The figure shows three views and two pictorial views of one solid part (mm, origin at its lowest corner). Answer the questions. Round coordinates to 2 decimals unless told otherwise and drop trailing zeros. Order: outer loops, then holes, each group sorted by start corner. A loop starts at its lowest first (then second) coordinate and runs counter-clockwise, first axis right, second up. Notation, with made-up numbers: (-19, 6) -> (19, 6) arc R33 ccw to (19, 36) -> close; hole circle Ø9 at (17, -28.75). An arc over 180 degrees is marked (long way). Return JSON: item names as keys, results as strings. Group by question number.
(1) Consider line 1 (X direction, y = 67, z = 2.4); line 2 (X direction, y = 86, z = 1.65). Determine where each line is inside the solid, lowest interval first. Write a range as [from, to].
(2) The part is cut by section B-B (y = 67). Determine the outline of the cut face in (x, z), plus the area to 3 significant figures.
(3) This flat-tipped pin is pushed along its axis until it touches: pin 1 (2.5 mm diameter, centred on x = 81, y = 67, fed in from -Z). Where does it stop, or does it pass through?
(4) The part is cut by section A-A (y = 126.5). Determine the outline of the cut face in (x, z), plus the area to 3 significant figures.
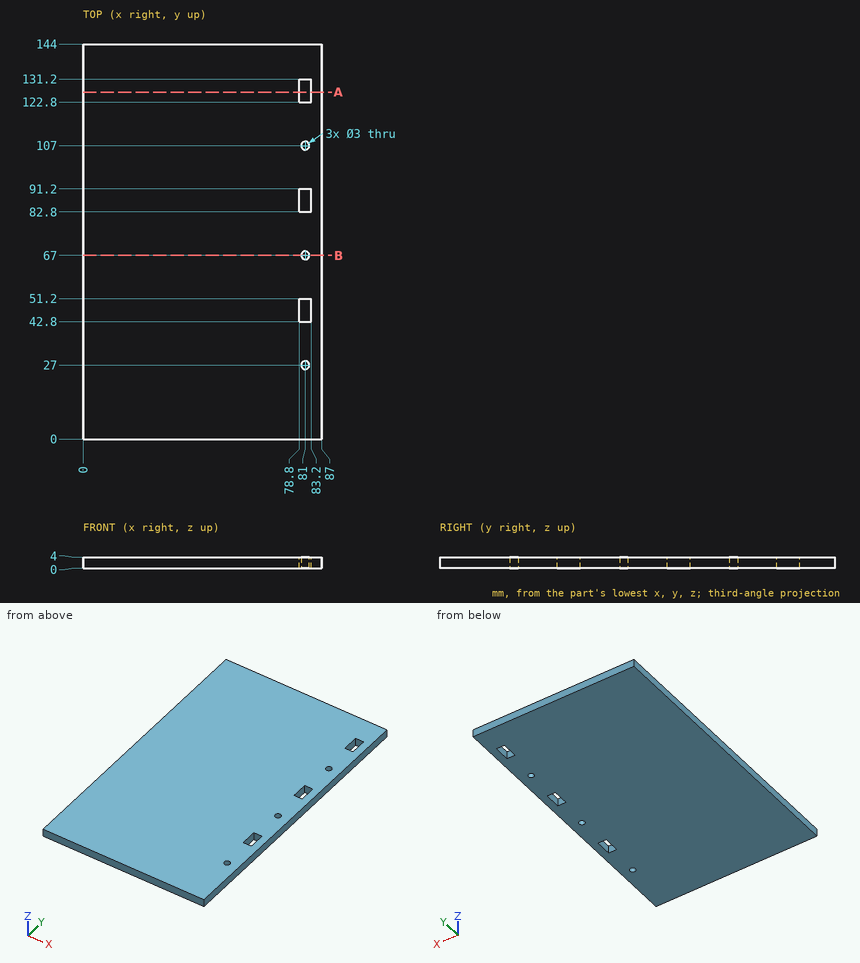
Answer below:
{
 "1": {"line 1": "x = [0, 79.5], [82.5, 87]", "line 2": "x = [0, 78.8], [83.2, 87]"},
 "2": {"outline": "(0, 0) -> (79.5, 0) -> (79.5, 4) -> (0, 4) -> close; (82.5, 0) -> (87, 0) -> (87, 4) -> (82.5, 4) -> close", "area": "336 mm²"},
 "3": {"pin 1": "passes through"},
 "4": {"outline": "(0, 0) -> (78.8, 0) -> (78.8, 4) -> (0, 4) -> close; (83.2, 0) -> (87, 0) -> (87, 4) -> (83.2, 4) -> close", "area": "330 mm²"}
}
